Check sheet for the modelled part. Datum: model origin and axes. Units: mm. A direction names the side the tool comes from. Round coordinates to 2 decimals unless told otherwise and drop trailing zeros. Write each loop counter-clockwise with the first axis right and the second up, starting at its lowest first coordinate (ties: lowest second). Pieces come first, ordered by that corner, then holes. Notation, with made-up numbers: (36.25, 68.25) - (40.25, 68.25) arc R23 ccw to (40.25, 105.25) - close; hole circle Ø10 at (74, 68.25). An arc over 180 degrees is marked (long way). Answer as a JSON object with one key per item and string values. Group by question number.
Item 1: Sectioned sample at A-A on y = 0. Record the boundary of the cut face in (x, z).
Item 2: Set-up check for faces 1 (the cylindrical face through (10.912, 83.107, -33.269)), 2 (the cylindrical face through (4.1, 91.17, -25.04)), 3 (the cylindrical face through (-99.79, 5.46, -21.91)), 4 (the flat face through (0, -8, 19.05)): record each of +Z, -Z, +X, -X, +Y, -Y from which the full face is reachable in a straight line by a thin tool's end or side.
Item 3: Release check for a two-part mould opening along Y. For faces 5 (the cylindrical face through (-3.85, -17.36, 22.27)), 6 (the cylindrical face through (111.445, 35.096, -25.044)), 7 (the cylindrical face through (76.907, -49.139, -25.044)), 8 (the flat face through (13, -13, 25.4)) record: pulls with the +Y half, pulls with the -Y half, needs draft (parallel to the pull), parting line crosses it, or undercut.
Item 4: Gauge pin test, flat ends, axial feed: P1, Ø10, axis at x = -19, y = 30.5, coming from the +Z side; P2, Ø6, axis at x = -21.5, z = -34.5, coming from the +Y side; P3, Ø5, axis at y = -10.5, z = -17.5, coming from the -X side. Record the tip position at first contact, or that the pin passes through.
Item 5: Sectioned sample at D-D on z = -30.48. Record the boundary of the cut face in (x, y).
Item 6: Sectioned sample at C-C on y = -99.06. Record the boundary of the cut face in (x, z), plus the area to 3 significant figures.
Item 7: Thickness scan on line 1 (X direction, y = 49, z = -13); line 2 (X direction, y = -57, z = -35); line 3 (X direction, y = 49, z = -16). Record the ranges inside material, lowest first.
Item 8: Sectioned sample at B-B on x = 0. Record the boundary of the cut face in (y, z).
Autodesk Inventor part; units mm, degrees
ref_plane "YZ Plane" through (0, 0, 0) normal (1, 0, 0) x (0, 1, 0)
ref_plane "XZ Plane" through (0, 0, 0) normal (0, 1, 0) x (-1, 0, 0)
ref_plane "XY Plane" through (0, 0, 0) normal (0, 0, 1) x (1, 0, 0)
sketch "Sketch1" plane through (0, 0, 0) normal (0, 0, 1) x (1, 0, 0)
  circle A0 centre (0, 0) radius 116.84
  circle A1 centre (0, 0) radius 30.48
  dimension "d0" = 233.68
  dimension "d1" = 60.96
extrude "Extrusion1" add sketch "Sketch1" against normal blind 50.8 contours A0 | A1
sketch "Sketch2" plane through (0, 0, 0) normal (0, 0, 1) x (1, 0, 0)
  circle A0 centre (0, 0) radius 30.48
  dimension "d4" = 60.96
extrude "Extrusion2" add sketch "Sketch2" along normal blind 25.4
sketch "Sketch3" plane through (0, 0, 25.4) normal (0, 0, 1) x (1, 0, 0)
  point P0 (0, 0)
sketch "Sketch4" plane through (0, 0, 25.4) normal (0, 0, 1) x (1, 0, 0)
  circle A0 centre (0, 0) radius 6.35
  circle A1 centre (0, 0) radius 17.78
  dimension "d7" = 12.7
  dimension "d8" = 35.56
extrude "Extrusion3" cut sketch "Sketch4" against normal blind 6.35 contours A0 | A1
extrude "Extrusion6" cut sketch "Sketch4" against normal through all contours A0
sketch "Sketch5" plane through (0, 0, -50.8) normal (0, 0, -1) x (-1, 0, 0)
  circle A0 centre (0, 0) radius 6.35
  circle A1 centre (0, 0) radius 83.82
  dimension "d17" = 167.64
extrude "Extrusion7" cut sketch "Sketch5" against normal blind 35.56
sketch "Sketch7" plane through (0, 0, 0) normal (1, 0, 0) x (0, 1, 0)
  circle A0 centre (0, -30.48) radius 10.16
  line L0 (-116.84, -50.8) -> (116.84, -50.8)
  point P0 (0, 0)
  dimension "d20" = 20.32
  dimension "d21" = 20.32
extrude "Extrusion8" cut sketch "Sketch7" against normal through all
thread "Thread1"
sketch "Sketch8" plane through (0, 0, 0) normal (0, 0, 1) x (1, 0, 0)
  point P0 (0, 0)
sketch "Sketch9" plane through (0, 0, 0) normal (0, 0, 1) x (1, 0, 0)
  circle A0 centre (0, 0) radius 6.35 construction
  circle A1 centre (0, 0) radius 99.06 construction
  line L0 (0, 0) -> (-123.6027, 71.3621) construction
  line L1 (0, 0) -> (-132.0824, -76.2578) construction
  line L2 (-189.6994, 0) -> (167.9299, 0) construction
  circle A2 centre (-85.7885, 49.53) radius 8.89
  circle A3 centre (-85.7885, -49.53) radius 8.89
  circle A4 centre (0, -99.06) radius 8.89
  circle A5 centre (85.7885, -49.53) radius 8.89
  circle A6 centre (85.7885, 49.53) radius 8.89
  circle A7 centre (0, 99.06) radius 8.89
  dimension "d26" = 198.12
  dimension "d27" = 60
  dimension "d28" = 17.78
  dimension "d31" = 360
extrude "Extrusion9" cut sketch "Sketch9" against normal through all
thread "Thread2"
equation "\"BendRadius\" = Thickness"
equation "\"BendReliefWidth\" = Thickness"
equation "\"BendReliefDepth\" = 0.5 * Thickness"
equation "\"CornerReliefSize\" = 4 * Thickness"
equation "\"MinimumRemnant\" = 2 * Thickness"
equation "\"TransitionRadius\" = BendRadius"
equation "\"JacobiRadiusSize\" = BendRadius"
equation "\"GapSize\" = Thickness"
properties part number "valve housing" material "Aluminum 6061"
Completed:
{
 "1": {"outline": "(-116.84, -50.8) - (-83.82, -50.8) - (-83.82, -40.64) - (-116.84, -40.64) - close; (-116.84, -20.32) - (-83.82, -20.32) - (-83.82, -15.24) - (-6.35, -15.24) - (-6.35, 19.05) - (-17.78, 19.05) - (-17.78, 25.4) - (-30.48, 25.4) - (-30.48, 0) - (-116.84, 0) - close; (6.35, -15.24) - (83.82, -15.24) - (83.82, -50.8) - (116.84, -50.8) - (116.84, 0) - (30.48, 0) - (30.48, 25.4) - (17.78, 25.4) - (17.78, 19.05) - (6.35, 19.05) - close"},
 "2": {"face 1": "-Z", "face 2": "+Z, -Z", "face 3": "-X", "face 4": "+Z"},
 "3": {"face 5": "undercut", "face 6": "parting line crosses it", "face 7": "undercut", "face 8": "needs draft"},
 "4": {"P1": "z = 0", "P2": "y = 115.37", "P3": "x = -116.57"},
 "5": {"outline": "(-116.4, -10.16) arc R116.84 ccw (long way) to (-116.4, 10.16) - (-83.2, 10.16) arc R83.82 cw (long way) to (-83.2, -10.16) - close; hole circle Ø17.78 at (-85.79, -49.53); hole circle Ø17.78 at (-85.79, 49.53); hole circle Ø17.78 at (0, -99.06); hole circle Ø17.78 at (0, 99.06); hole circle Ø17.78 at (85.79, -49.53); hole circle Ø17.78 at (85.79, 49.53)"},
 "6": {"outline": "(-61.96, -50.8) - (-8.89, -50.8) - (-8.89, 0) - (-61.96, 0) - close; (8.89, -50.8) - (61.96, -50.8) - (61.96, 0) - (8.89, 0) - close", "area": "5,390 mm²"},
 "7": {"line 1": "-106.07 to -94.66, -76.91 to 76.91, 94.66 to 106.07", "line 2": "-101.99 to -90.61, -80.97 to -61.46, 61.46 to 80.97, 90.61 to 101.99", "line 3": "-106.07 to -94.66, -76.91 to -68.01, 68.01 to 76.91, 94.66 to 106.07"},
 "8": {"outline": "(-116.84, -50.8) - (-107.95, -50.8) - (-107.95, 0) - (-116.84, 0) - close; (-90.17, -50.8) - (-83.82, -50.8) - (-83.82, -15.24) - (-6.35, -15.24) - (-6.35, 19.05) - (-17.78, 19.05) - (-17.78, 25.4) - (-30.48, 25.4) - (-30.48, 0) - (-90.17, 0) - close; (6.35, -15.24) - (83.82, -15.24) - (83.82, -50.8) - (90.17, -50.8) - (90.17, 0) - (30.48, 0) - (30.48, 25.4) - (17.78, 25.4) - (17.78, 19.05) - (6.35, 19.05) - close; (107.95, -50.8) - (116.84, -50.8) - (116.84, 0) - (107.95, 0) - close"}
}
